Check sheet for the modelled part. Datum: model origin and axes. Units: mm. Face numbers are marked on the shaded views. A direction names the side the tool comes from. Round coordinates to 2 decimals unless told otherwise and drop trailing zeros. Loops run counter-clockwise (first coordinate to the right, second up) from the corner with the lowest first, then second, coordinate; pieces in that order, holes last. Notation, with made-up numbers: (60, 2.25) - (114, 2.25) arc R17 cw to (114, 20.25) - close; hole circle Ø1 at (15.5, 21). An arc over 180 degrees is marked (long way). Return JSON: item names as keys, results as strings.
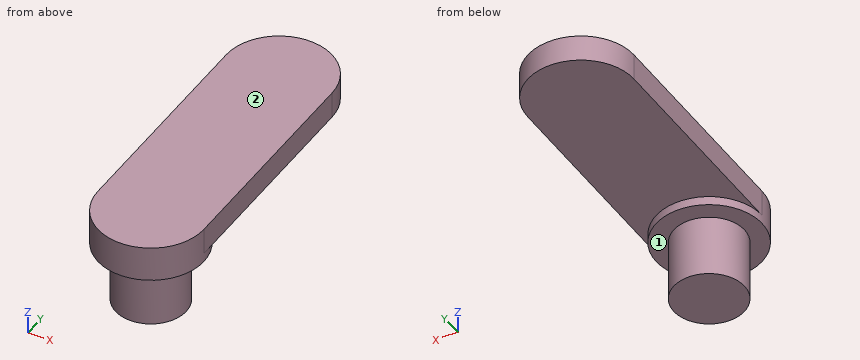
from build123d import *

# Parameters (mm, degrees)
SKETCH1_R           = 6
BOSS_EXTRUDE1_DEPTH = 1
BOSS_EXTRUDE2_DEPTH = 3
SKETCH3_R           = 4
BOSS_EXTRUDE3_DEPTH = 7


with BuildPart() as part:
    # Sketch1 → Boss-Extrude1 (new body)
    with BuildSketch(Plane.XY):
        Circle(SKETCH1_R)
    extrude(amount=-BOSS_EXTRUDE1_DEPTH)

    # Sketch2 → Boss-Extrude2 (add)
    with BuildSketch(Plane.XY):
        with BuildLine():
            Line((-6, 0), (-6, 25))
            ThreePointArc((-6, 25), (0, 31), (6, 25))
            Line((6, 25), (6, 0))
            ThreePointArc((6, 0), (0, -6), (-6, 0))
        make_face()
    extrude(amount=BOSS_EXTRUDE2_DEPTH)

    # Sketch3 → Boss-Extrude3 (add)
    with BuildSketch(Plane(origin=(0, 0, -1), x_dir=(-1, 0, 0), z_dir=(0, 0, -1))):
        Circle(SKETCH3_R)
    extrude(amount=BOSS_EXTRUDE3_DEPTH)


solid = part.part
Q1. Scan lines: probe 1 along Z at (x, y) = (2.5, 23.5); probe 2 along Y at (x, z) = (-0.25, -2); probe 3 along Y at (x, z) = (1.75, -4.75). Record each from-to range of solid material in increasing order. Write a range as [from, to].
Answer key:
{"probe 1": "z = [0, 3]", "probe 2": "y = [-3.99, 3.99]", "probe 3": "y = [-3.6, 3.6]"}
Q2. Sectioned sample at D-D (x = 3). Enter the section's corners in (y, z).
Answer key:
{"outline": "(-5.2, -1) - (-2.65, -1) - (-2.65, -8) - (2.65, -8) - (2.65, -1) - (5.2, -1) - (5.2, 0) - (30.2, 0) - (30.2, 3) - (-5.2, 3) - close"}
Q3. Sectioned sample at C-C (y = 21). Enter the section's corners in (x, z), plus the area to 3 significant figures.
Answer key:
{"outline": "(-6, 0) - (6, 0) - (6, 3) - (-6, 3) - close", "area": "36.0 mm²"}
Q4. Depth check by flat-ended pin: P1, Ø5, axis at x = -1.5, y = 24.5, coming from the -Z side; P2, Ø1, axis at x = -1.5, z = -1, coming from the -Y side; P3, Ø5, axis at x = 2, z = -4.5, coming from the +Y side; P4, Ø1.5, axis at y = 5, z = -6, coming from the +X side. Enter the tip coordinate at first touch or a pass-through.
Answer key:
{"P1": "stops at z = 0", "P2": "stops at y = -5.92", "P3": "stops at y = 4", "P4": "passes through"}
Q5. Tool access check on the marked faces 1 and 2. Record the directions out of +Z, -Z, +X, -X, +Y, -Y that give a thin tool (end or side, any length) a straight path to the whole face; none if there is none.
Answer key:
{"face 1": "-Z", "face 2": "+Z, +X, -X, +Y, -Y"}
Q6. Sectioned sample at A-A (x = 0). Enter the section's corners in (y, z), plus the area to 3 significant figures.
Answer key:
{"outline": "(-6, -1) - (-4, -1) - (-4, -8) - (4, -8) - (4, -1) - (6, -1) - (6, 0) - (31, 0) - (31, 3) - (-6, 3) - close", "area": "179 mm²"}
Q7. Sectioned sample at B-B (z = 2). Enter the section's corners in (x, y).
Answer key:
{"outline": "(-6, 0) arc R6 ccw to (6, 0) - (6, 25) arc R6 ccw to (-6, 25) - close"}
